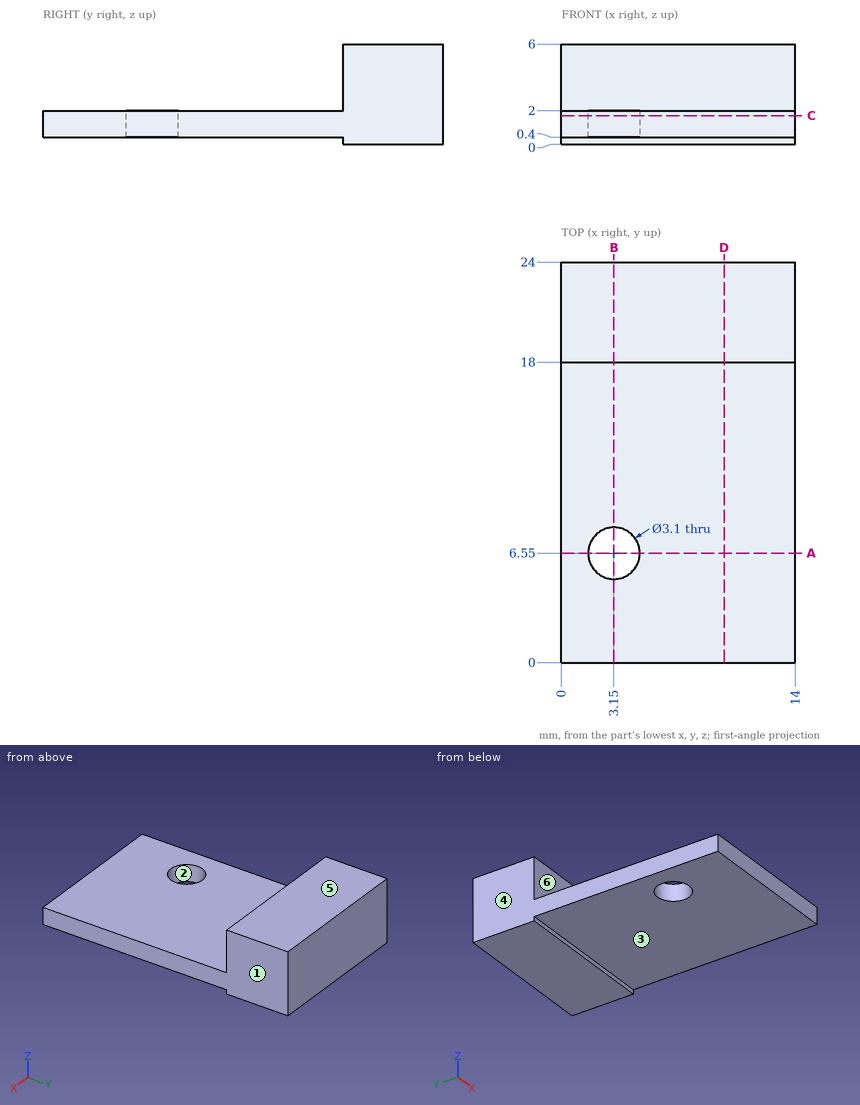
Verification items for this drawing (mm, ordinates from the low corner). A direction names the side the tool comes from. Give positions to 0.01 mm unless a question says otherwise; leave off trailing zeros. Order: outer loops, then holes, each group sorted by start corner. A loop starts at its lowest first (then second) coordinate and runs counter-clockwise, first axis right, second up.
1) Cross-section at B-B (x = 3.15). Record the boundary of the cut face in (y, z), then the cut area to 3 significant figures.
Results are:
outline: (0, 0.4) - (5, 0.4) - (5, 2) - (0, 2) - close; (8.1, 0.4) - (18, 0.4) - (18, 0) - (24, 0) - (24, 6) - (18, 6) - (18, 2) - (8.1, 2) - close
area: 59.8 mm2
2) Draft check along X on the marked faces 1, 2, 3 and 4. Enter one of: released by +X, released by -X, zero draft, split by the parting line, or undercut.
Results are:
face 1: released by +X
face 2: undercut
face 3: zero draft
face 4: released by -X
3) Material ranges on probe 1 along Y at (x, z) = (3.15, 1.15); probe 2 along Z at (x, y) = (1.25, 5.75); probe 3 along Y at (x, z) = (9.75, 4.1), recorded low to high.
Results are:
probe 1: y = 0 to 5, 8.1 to 24
probe 2: z = 0.4 to 2
probe 3: y = 18 to 24
4) Tool access check on the marked faces 5 and 6. Record the directions out of +Z, -Z, +X, -X, +Y, -Y that give a thin tool (end or side, any length) a straight path to the whole face; none if there is none.
Results are:
face 5: +Z, +X, -X, +Y, -Y
face 6: +Z, +X, -X, -Y
5) Cross-section at C-C (z = 1.7). Record the boundary of the cut face in (x, y).
Results are:
outline: (0, 0) - (14, 0) - (14, 24) - (0, 24) - close; hole circle Ø3.1 at (3.15, 6.55)
6) Cross-section at A-A (y = 6.55). Record the boundary of the cut face in (x, z), then the cut area to 3 significant figures.
Results are:
outline: (0, 0.4) - (1.6, 0.4) - (1.6, 2) - (0, 2) - close; (4.7, 0.4) - (14, 0.4) - (14, 2) - (4.7, 2) - close
area: 17.4 mm2
7) Gauge pin test, flat ends, axial feed: pin 1 (5 mm diameter, centred on x = 6.5, y = 5.5, fed in from +Z); pin 2 (2 mm diameter, centred on x = 3.5, z = 4.5, fed in from -Y); pin 3 (6 mm diameter, centred on x = 6.5, y = 7, fed in from -Z). Record the tip position at first contact, or that the pin passes through.
Results are:
pin 1: stops at z = 2
pin 2: stops at y = 18
pin 3: stops at z = 0.4
8) Cross-section at D-D (x = 9.75). Record the boundary of the cut face in (y, z), then the cut area to 3 significant figures.
Results are:
outline: (0, 0.4) - (18, 0.4) - (18, 0) - (24, 0) - (24, 6) - (18, 6) - (18, 2) - (0, 2) - close
area: 64.8 mm2
